Design review of the part built by this model. Coordinates are the model's own, in mm. A direction names the side the tool comes from. Give positions to 0.01 mm unless a question says otherwise; leave off trailing zeros. Loops run counter-clockwise (first coordinate to the right, second up) from the corner with the lowest first, then second, coordinate; pieces in that order, holes last. Notation, with made-up numbers: M 48.25,41.5 L 94.25,41.5 A9 cw 94.25,54.5 Z; hole C 28,0 d9. An arc over 180 degrees is marked long. Use CSV: the item, a comma, the result in double quotes.
from build123d import *

# Parameters (mm, degrees)
SKETCH1_R           = 10.5
BOSS_EXTRUDE1_DEPTH = 26
BOSS_EXTRUDE2_START = 26
SKETCH1_3_R         = 19
BOSS_EXTRUDE2_DEPTH = 3
BOSS_EXTRUDE3_START = 29
SKETCH1_4_R         = 10.5
BOSS_EXTRUDE3_DEPTH = 100
BOSS_EXTRUDE4_START = 129
SKETCH1_5_R         = 19
BOSS_EXTRUDE4_DEPTH = 3
BOSS_EXTRUDE5_START = 132
SKETCH1_6_R         = 10.5
BOSS_EXTRUDE5_DEPTH = 52
CHAMFER1_SIZE       = 2


with BuildPart() as part:
    # Sketch1 → Boss-Extrude1 (new body)
    with BuildSketch(Plane(origin=(0, 0, 0), x_dir=(1, 0, 0), z_dir=(0, 1, 0))):
        Circle(SKETCH1_R)
    extrude(amount=BOSS_EXTRUDE1_DEPTH)

    # Sketch1<3> → Boss-Extrude2 (add)
    with BuildSketch(Plane(origin=(0, 0, 0), x_dir=(1, 0, 0), z_dir=(0, 1, 0)).offset(BOSS_EXTRUDE2_START)):
        Circle(SKETCH1_3_R)
    extrude(amount=BOSS_EXTRUDE2_DEPTH)

    # Sketch1<4> → Boss-Extrude3 (add)
    with BuildSketch(Plane(origin=(0, 0, 0), x_dir=(1, 0, 0), z_dir=(0, 1, 0)).offset(BOSS_EXTRUDE3_START)):
        Circle(SKETCH1_4_R)
    extrude(amount=BOSS_EXTRUDE3_DEPTH)

    # Sketch1<5> → Boss-Extrude4 (add)
    with BuildSketch(Plane(origin=(0, 0, 0), x_dir=(1, 0, 0), z_dir=(0, 1, 0)).offset(BOSS_EXTRUDE4_START)):
        Circle(SKETCH1_5_R)
    extrude(amount=BOSS_EXTRUDE4_DEPTH)

    # Sketch1<6> → Boss-Extrude5 (add)
    with BuildSketch(Plane(origin=(0, 0, 0), x_dir=(1, 0, 0), z_dir=(0, 1, 0)).offset(BOSS_EXTRUDE5_START)):
        Circle(SKETCH1_6_R)
    extrude(amount=BOSS_EXTRUDE5_DEPTH)

    # Chamfer1
    chamfer1_edges = [part.edges().sort_by_distance(p)[0] for p in [
        (-10.5, 184, 0),
        (-10.5, 0, 0),
    ]]
    chamfer(chamfer1_edges, length=CHAMFER1_SIZE)


solid = part.part
(1) We need section D-D on y = 109. State the section outline as (x, z) points, then the cut area to 3 significant figures.
A:
outline,"C 0,0 d21"
area,"346 mm²"
(2) We need section A-A on z = 0. State the section outline as (x, y) points.
A:
outline,"M -19,26 L -10.5,26 L -10.5,2 L -8.5,0 L 8.5,0 L 10.5,2 L 10.5,26 L 19,26 L 19,29 L 10.5,29 L 10.5,129 L 19,129 L 19,132 L 10.5,132 L 10.5,182 L 8.5,184 L -8.5,184 L -10.5,182 L -10.5,132 L -19,132 L -19,129 L -10.5,129 L -10.5,29 L -19,29 Z"
(3) We need section B-B on x = 0. State the section outline as (y, z) points.
A:
outline,"M 0,-8.5 L 2,-10.5 L 26,-10.5 L 26,-19 L 29,-19 L 29,-10.5 L 129,-10.5 L 129,-19 L 132,-19 L 132,-10.5 L 182,-10.5 L 184,-8.5 L 184,8.5 L 182,10.5 L 132,10.5 L 132,19 L 129,19 L 129,10.5 L 29,10.5 L 29,19 L 26,19 L 26,10.5 L 2,10.5 L 0,8.5 Z"
(4) We need section C-C on z = -12.5. State the section outline as (x, y) points, then the cut area to 3 significant figures.
A:
outline,"M -14.31,26 L 14.31,26 L 14.31,29 L -14.31,29 Z; M -14.31,129 L 14.31,129 L 14.31,132 L -14.31,132 Z"
area,"172 mm²"
(5) Clearance check with flat-ended pins moving along their axes: P1, Ø12, axis at x = -3.5, y = 88.5, coming from the -Z side; P2, Ø1.5, axis at x = -5, y = 137.5, coming from the +Z side; P3, Ø1, axis at x = -13, z = -9.5, coming from the -Y side. State where each tip first meets the part, or that it passes through.
A:
P1,"z = -10.5"
P2,"z = 9.6"
P3,"y = 26"
(6) Machinability: for faces 4 (the cylindrical face through (10, 156.6, -3.2)), 5 (the flat face through (8, 29, 8)), 6 (the flat face through (8, 26, 8)), which of the approach directions +Z, -Z, +X, -X, +Y, -Y give a long, thin tool a straight path to every point of the face, cutting with its end or side? Answer none if there is none.
A:
face 4,"+Y"
face 5,"none"
face 6,"-Y"
(7) Wall thickness on line 1 along Y through (x, z) = (-6, 16.5); line 2 along Z through (x, y) = (-0.5, 155); line 3 along X through (y, z) = (59, 9): over which ranges is each line inside the solid? List them lowest first. Write a range as [from, to].
A:
line 1,"[26, 29], [129, 132]"
line 2,"[-10.49, 10.49]"
line 3,"[-5.41, 5.41]"
(8) The part is to be moulded in two halves that separate along Y. For faces 1 (the cylindrical face through (10, 78.3, -3.2)), 2 (the cylindrical face through (10, 13.8, -3.2)), 3 (the flat face through (0, 184, 0)), say which applies: released by +Y, released by -Y, zero draft, split by the parting line, or undercut.
A:
face 1,"undercut"
face 2,"zero draft"
face 3,"released by +Y"
